from build123d import *

# Parameters (mm, degrees)
F1_DEPTH = 3


with BuildPart() as f1:
    # F0 (on Front) → F1 (new body)
    with BuildSketch(Plane.XZ):
        with BuildLine():
            Line((27.675254, 25.977628), (-32.324746, 25.977628))
            ThreePointArc((-32.324746, 25.977628), (-36.290467, 25.580511), (-40.098703, 24.404933))
            Line((-40.098703, 24.404933), (-40.098703, 19.404933))
            Line((-40.098703, 19.404933), (-42.767557, 19.404933))
            Line((-42.767557, 19.404933), (-42.767557, 23.034817))
            ThreePointArc((-42.767557, 23.034817), (-49.772614, 15.753715), (-52.324746, 5.977628))
            Line((-52.324746, 5.977628), (-52.324746, 0.977628))
            ThreePointArc((-52.324746, 0.977628), (-46.466882, -13.164508), (-32.324746, -19.022372))
            Line((-32.324746, -19.022372), (-32.324746, -9.022372))
            Line((-32.324746, -9.022372), (-29.324746, -9.022372))
            Line((-29.324746, -9.022372), (-29.324746, -19.022372))
            Line((-29.324746, -19.022372), (24.675254, -19.022372))
            Line((24.675254, -19.022372), (24.675254, -9.022372))
            Line((24.675254, -9.022372), (27.675254, -9.022372))
            Line((27.675254, -9.022372), (27.675254, -19.022372))
            ThreePointArc((27.675254, -19.022372), (41.81739, -13.164508), (47.675254, 0.977628))
            Line((47.675254, 0.977628), (47.675254, 5.977628))
            ThreePointArc((47.675254, 5.977628), (46.674828, 12.223921), (43.773636, 17.845318))
            Line((43.773636, 17.845318), (40.629784, 14.421898))
            Line((40.629784, 14.421898), (38.435426, 16.437057))
            Line((38.435426, 16.437057), (41.81739, 20.119763))
            ThreePointArc((41.81739, 20.119763), (35.328923, 24.455218), (27.675254, 25.977628))
        make_face()
    extrude(amount=F1_DEPTH)


solid = f1.part
Source: CAD feature listing. Evaluate the final solid. Frame: model axes, mm. A direction names the side the tool comes from. Give positions to 0.01 mm unless a question says otherwise; leave off trailing zeros. Order: outer loops, then holes, each group sorted by start corner. A loop starts at its lowest first (then second) coordinate and runs counter-clockwise, first axis right, second up. Notation, with made-up numbers: (87.25, 17.25) -> (136.25, 17.25) arc R21 ccw to (136.25, 36.25) -> close; hole circle Ø4 at (23.5, 35). An arc over 180 degrees is marked (long way). Use a Markdown table: item, result.
1) Section query B-B, the plane y = -2.4. Return the cut outline in (x, z), then the cut area to 3 significant figures.
Answer list:
| item | result |
|---|---|
| outline | (-52.32, 0.98) arc R20 ccw to (-32.32, -19.02) -> (-32.32, -9.02) -> (-29.32, -9.02) -> (-29.32, -19.02) -> (24.68, -19.02) -> (24.68, -9.02) -> (27.68, -9.02) -> (27.68, -19.02) arc R20 ccw to (47.68, 0.98) -> (47.68, 5.98) arc R20 ccw to (43.77, 17.85) -> (40.63, 14.42) -> (38.44, 16.44) -> (41.82, 20.12) arc R20 ccw to (27.68, 25.98) -> (-32.32, 25.98) arc R20 ccw to (-40.1, 24.4) -> (-40.1, 19.4) -> (-42.77, 19.4) -> (-42.77, 23.03) arc R20 ccw to (-52.32, 5.98) -> close |
| area | 4,070 mm² |
2) Ray query, line 1 along X through (y, z) = (-0.4, -13); line 2 along X through (y, z) = (-0.45, -11.5); line 3 along Z through (x, y) = (28.5, -1.3). Return the intervals inside material, ascending. Write a range as [from, to].
Answer list:
| item | result |
|---|---|
| line 1 | [-46.63, -32.32], [-29.32, 24.68], [27.68, 41.98] |
| line 2 | [-47.96, -32.32], [-29.32, 24.68], [27.68, 43.31] |
| line 3 | [-19.01, 25.96] |
3) Section query A-A, the plane z = -15.5. Return the cut outline in (x, y), then the cut area to 3 significant figures.
Answer list:
| item | result |
|---|---|
| outline | (-43.66, -3) -> (-32.32, -3) -> (-32.32, 0) -> (-43.66, 0) -> close; (-29.32, -3) -> (24.68, -3) -> (24.68, 0) -> (-29.32, 0) -> close; (27.68, -3) -> (39.01, -3) -> (39.01, 0) -> (27.68, 0) -> close |
| area | 230 mm² |
4) Section query C-C, the plane x = -38. Return the cut outline in (y, z), then the cut area to 3 significant figures.
Answer list:
| item | result |
|---|---|
| outline | (-3, -18.2) -> (0, -18.2) -> (0, 25.16) -> (-3, 25.16) -> close |
| area | 130 mm² |
5) Section query D-D, the plane z = -5. Return the cut outline in (x, y).
Answer list:
| item | result |
|---|---|
| outline | (-51.41, -3) -> (46.76, -3) -> (46.76, 0) -> (-51.41, 0) -> close |
6) Reachability of faces 5 (the flat face through (-31, -1, -9.022)), 6 (the flat face through (40.1, -1.48, 18.25)), 7 (the flat face through (-52.325, -1, 4)), 8 (the flat face through (-42.768, -1, 21)), 9 (the flat face through (-3, -1, -19.022)) from +Z, -Z, +X, -X, +Y, -Y: full face, straight path, thin tool, end or side. Return the list, or none.
Answer list:
| item | result |
|---|---|
| face 5 | -Z, +Y, -Y |
| face 6 | +Y, -Y |
| face 7 | +Z, -Z, -X, +Y, -Y |
| face 8 | +Z, +Y, -Y |
| face 9 | -Z, +X, -X, +Y, -Y |
7) Mould query, pull axis X, two halves, no side actions, for faces 1 (the flat face through (27.675, -1, -14)), 2 (the cylindrical face through (41.66, -1.48, -13.32)), 3 (the flat face through (24.675, -1, -14)), 4 (the flat face through (-2, -1, 25.978)). Classes: +X half, -X half, draft (parallel to the pull), parting line (faces both ways), or undercut.
Answer list:
| item | result |
|---|---|
| face 1 | undercut |
| face 2 | +X half |
| face 3 | undercut |
| face 4 | draft |
8) Contact query for flat-ended pins moving along their axis: P1, Ø1.5, axis at x = -31, y = -1, coming from the -Z side; P2, Ø1.5, axis at y = -1.5, z = -11.5, coming from the -X side; P3, Ø1, axis at y = -2.5, z = -14.5, coming from the +X side. Output: stop coordinate, or through.
Answer list:
| item | result |
|---|---|
| P1 | z = -9.02 |
| P2 | x = -48.53 |
| P3 | x = 40.93 |
